```python
from build123d import *

# Parameters (mm, degrees)
CROQUIS1_R                   = 67.818
CROQUIS1_R_2                 = 18.923
SALIENTE_EXTRUIR1_DEPTH      = 50
CORPS_D_PLACER_COPIER1_ANGLE = 90


with BuildPart() as part:
    # Croquis1 → Saliente-Extruir1 (new body)
    with BuildSketch(Plane.XY):
        with BuildLine():
            Line((50.841156462, -86.860973253), (100.076, -8.434146427))
            Line((100.076, -8.434146427), (100.076, 106.373853573))
            ThreePointArc((100.076, 106.373853573), (0, 146.05), (-100.076, 106.373853573))
            Line((-100.076, 106.373853573), (-100.076, -8.434146427))
            Line((-100.076, -8.434146427), (-51.520843538, -86.217090682))
            Line((-51.520843538, -86.217090682), (-51.520843538, -312.023090682))
            ThreePointArc((-51.520843538, -312.023090682), (-0.468123725, -332.738527707), (50.841156462, -312.666973253))
            Line((50.841156462, -312.666973253), (50.841156462, -86.860973253))
        make_face()
        Circle(CROQUIS1_R, mode=Mode.SUBTRACT)
        with Locations((0, -296.418)):
            Circle(CROQUIS1_R_2, mode=Mode.SUBTRACT)
        with BuildLine():
            Line((18.923, -116.332), (18.923, -227.838))
            ThreePointArc((18.923, -227.838), (0, -246.761), (-18.923, -227.838))
            Line((-18.923, -227.838), (-18.923, -116.332))
            ThreePointArc((-18.923, -116.332), (0, -97.409), (18.923, -116.332))
        make_face(mode=Mode.SUBTRACT)
    extrude(amount=SALIENTE_EXTRUIR1_DEPTH)


with BuildPart() as part_1:
    # Corps-Déplacer/Copier1: moved
    add(part.part.rotate(Axis((0, 0, 0), (0, 0, 1)), CORPS_D_PLACER_COPIER1_ANGLE))


solid = part_1.part
```
The listing builds one solid part. Answer for the finished solid, in the listing's coordinates (mm). A direction names the side the tool comes from. Coordinates: 2 decimals unless noted, no trailing zeros. Write each loop counter-clockwise with the first axis right and the second up, starting at its lowest first coordinate (ties: lowest second). Pieces come first, ordered by that corner, then holes. Notation, with made-up numbers: (78, 33) - (89, 33) arc R10 cw to (89, 50) - close; hole circle Ø2 at (76.5, 35). An arc over 180 degrees is marked (long way). One line per item, written item: value.
1) Find section C-C (z = 15.5). Give the vertices of the cut face in (x, y), and give its area (3 significant figures).
Geometry check:
outline: (-106.37, -100.08) - (8.43, -100.08) - (86.22, -51.52) - (312.02, -51.52) arc R74.42 ccw to (312.67, 50.84) - (86.86, 50.84) - (8.43, 100.08) - (-106.37, 100.08) arc R146.05 ccw to start; hole circle Ø135.64 at (0, 0); hole (116.33, -18.92) - (227.84, -18.92) arc R18.92 ccw to (227.84, 18.92) - (116.33, 18.92) arc R18.92 ccw to start; hole circle Ø37.85 at (296.42, 0)
area: 43,900 mm2
2) Each of these flat-tipped pins is pushed along its axis until it touches: pin 1 Ø10 at (y, z) = (-29.5, 26.5) entering from +X; pin 2 Ø1 at (y, z) = (-66.5, 9.5) entering from -X; pin 3 Ø12 at (y, z) = (-13, 12) entering from -X. Where does it stop, or does it pass through?
Geometry check:
pin 1: stops at x = 328.59
pin 2: stops at x = -130.29
pin 3: stops at x = -145.88
3) For a pull along Y with two mould halves and no side action, classify faces 1 (the flat face through (173, -18.923, 25)), 2 (the flat face through (48.2, 75.11, 24.65)), 3 (the flat face through (198, -51.521, 25)), 4 (the flat face through (90, -1, 50)) as pulls with the +Y half, pulls with the -Y half, needs draft (parallel to the pull), parting line crosses it, or undercut.
Geometry check:
face 1: undercut
face 2: pulls with the +Y half
face 3: pulls with the -Y half
face 4: needs draft
4) Find section A-A (y = 0). Give the vertices of the cut face in (x, z) (3 decimals).
Geometry check:
outline: (-146.05, 0) - (-67.818, 0) - (-67.818, 50) - (-146.05, 50) - close; (67.818, 0) - (97.409, 0) - (97.409, 50) - (67.818, 50) - close; (246.761, 0) - (277.495, 0) - (277.495, 50) - (246.761, 50) - close; (315.341, 0) - (332.74, 0) - (332.74, 50) - (315.341, 50) - close
5) Find section D-D (y = -60). Give the vertices of the cut face in (x, z).
Geometry check:
outline: (-133.16, 0) - (-31.61, 0) - (-31.61, 50) - (-133.16, 50) - close; (31.61, 0) - (72.63, 0) - (72.63, 50) - (31.61, 50) - close
6) Find section B-B (x = 0). Give the vertices of the cut face in (y, z).
Geometry check:
outline: (-100.08, 0) - (-67.82, 0) - (-67.82, 50) - (-100.08, 50) - close; (67.82, 0) - (100.08, 0) - (100.08, 50) - (67.82, 50) - close
7) A tool of negligible diameter and unlimited length cuts with its end or side. For faces 5 (the cylindrical face through (-146.04, 1.54, 24.65)), 6 (the flat face through (201, 50.841, 25)), 7 (the flat face through (171, 18.923, 25)), from which of +Z, -Z, +X, -X, +Y, -Y can it reach the whole face along a straight path? Write none if from no direction.
Geometry check:
face 5: +Z, -Z, -X
face 6: +Z, -Z, +X, +Y
face 7: +Z, -Z
8) Consider line 1 along X through (y, z) = (0, 28.5) (3 decimals); line 2 along X through (y, z) = (-14.5, 12.5); line 3 along Y through (x, z) = (197.5, 25). Determine where each line is inside the solid, lowest interval first. Write a range as from..to.
Geometry check:
line 1: x = -146.05..-67.818, 67.818..97.409, 246.761..277.495, 315.341..332.74
line 2: x = -145.33..-66.25, 66.25..104.17, 240..284.26, 308.58..331.31
line 3: y = -51.52..-18.92, 18.92..50.84
